Source: CAD feature listing. Evaluate the final solid. Frame: model axes, mm. A direction names the side the tool comes from. Coordinates: 2 decimals unless noted, no trailing zeros. Loops run counter-clockwise (first coordinate to the right, second up) from the corner with the lowest first, then second, coordinate; pieces in that order, holes last. Notation, with made-up numbers: (28, 24) -> (69, 24) arc R14 ccw to (69, 49) -> close; hole circle Ø9 at (77, 43.5). An arc over 180 degrees is marked (long way). Answer as CSV lines item,"result".
from build123d import *

# Parameters (mm, degrees)
SKETCH1_W          = 160
SKETCH1_H          = 70
EXTRUDE1_DEPTH     = 20
SKETCH2_W          = 40
SKETCH2_H          = 70
SKETCH2_W_2        = 20
SKETCH2_H_2        = 50
EXTRUDE2_DEPTH     = 10
SKETCH3_W          = 10
SKETCH3_H          = 10
CUT_EXTRUDE1_DEPTH = 1


with BuildPart() as part:
    # Sketch1 → Extrude1 (new body)
    with BuildSketch(Plane(origin=(0, 0, 0), x_dir=(1, 0, 0), z_dir=(0, 1, 0))):
        with Locations((80, 35)):
            Rectangle(SKETCH1_W, SKETCH1_H)
    extrude(amount=EXTRUDE1_DEPTH)

    # Sketch2 → Extrude2 (add)
    with BuildSketch(Plane(origin=(0, 20, 0), x_dir=(-1, 0, 0), z_dir=(0, 1, 0))):
        with Locations((-20, -35)):
            Rectangle(SKETCH2_W, SKETCH2_H)
        with Locations((-20, -35)):
            Rectangle(SKETCH2_W_2, SKETCH2_H_2, mode=Mode.SUBTRACT)
    extrude(amount=EXTRUDE2_DEPTH)

    # Sketch3 → Cut-Extrude1 (cut)
    with BuildSketch(Plane(origin=(0, 20, 0), x_dir=(-1, 0, 0), z_dir=(0, 1, 0))):
        with Locations((-110, -60)):
            Rectangle(SKETCH3_W, SKETCH3_H)
        with Locations((-110, -35)):
            Rectangle(SKETCH3_W, SKETCH3_H)
        with Locations((-135, -35)):
            Rectangle(SKETCH3_W, SKETCH3_H)
        with Locations((-60, -60)):
            Rectangle(SKETCH3_W, SKETCH3_H)
        with Locations((-60, -10)):
            Rectangle(SKETCH3_W, SKETCH3_H)
        with Locations((-135, -60)):
            Rectangle(SKETCH3_W, SKETCH3_H)
        with Locations((-135, -10)):
            Rectangle(SKETCH3_W, SKETCH3_H)
        with Locations((-110, -10)):
            Rectangle(SKETCH3_W, SKETCH3_H)
        with Locations((-85, -10)):
            Rectangle(SKETCH3_W, SKETCH3_H)
        with Locations((-85, -60)):
            Rectangle(SKETCH3_W, SKETCH3_H)
        with Locations((-60, -35)):
            Rectangle(SKETCH3_W, SKETCH3_H)
        with Locations((-85, -35)):
            Rectangle(SKETCH3_W, SKETCH3_H)
    extrude(amount=-CUT_EXTRUDE1_DEPTH, mode=Mode.SUBTRACT)


solid = part.part
(1) Draft query along X for faces 1 (the flat face through (110, 19, -10)), 2 (the flat face through (40, 25, -35)), 3 (the flat face through (81, 11, 0)). Return one class per face: released by +X, released by -X, zero draft, split by the parting line, or undercut.
Computed values:
face 1,"undercut"
face 2,"released by +X"
face 3,"zero draft"
(2) Cut plane A-A (y = 25.5). Return the cut outline in (x, z).
Computed values:
outline,"(0, -70) -> (40, -70) -> (40, 0) -> (0, 0) -> close; hole (10, -60) -> (30, -60) -> (30, -10) -> (10, -10) -> close"
(3) Cut plane C-C (x = 61). Return the cut outline in (y, z), then the cut area to 3 significant figures.
Computed values:
outline,"(0, -70) -> (20, -70) -> (20, -65) -> (19, -65) -> (19, -55) -> (20, -55) -> (20, -40) -> (19, -40) -> (19, -30) -> (20, -30) -> (20, -15) -> (19, -15) -> (19, -5) -> (20, -5) -> (20, 0) -> (0, 0) -> close"
area,"1,370 mm^2"
(4) Access query for faces 4 (the flat face through (60, 19, -10)), 5 (the flat face through (79, 0, -35)). Directions: +Z, -Z, +X, -X, +Y, -Y. A direction counts if a zero-diameter tool reaches every point of the face in a straight line with its end or side. Return the directions, or none.
Computed values:
face 4,"+Y"
face 5,"+Z, -Z, +X, -X, -Y"
(5) Material intervals for L1, parallel to Z at x = 61.5, y = 19.25; L2, parallel to X at y = 23.5, z = -24; L3, parallel to Z at x = 16.5, y = 22.75, sorted ascending. Write a range as [from, to].
Computed values:
L1,"[-70, -65], [-55, -40], [-30, -15], [-5, 0]"
L2,"[0, 10], [30, 40]"
L3,"[-70, -60], [-10, 0]"
(6) Cut plane B-B (z = -48). Return the cut outline in (x, y), then the cut area to 3 significant figures.
Computed values:
outline,"(0, 0) -> (160, 0) -> (160, 20) -> (40, 20) -> (40, 30) -> (30, 30) -> (30, 20) -> (10, 20) -> (10, 30) -> (0, 30) -> close"
area,"3,400 mm^2"
(7) Pin query (flat end, axial travel): pin 1 Ø1.1 at (y, z) = (19.5, -10) entering from -X; pin 2 Ø3 at (x, z) = (132.5, -21) entering from +Y. Return the tip coordinate at first contact, or that it passes through.
Computed values:
pin 1,"x = 0"
pin 2,"y = 20"
